from build123d import *

# Parameters (mm, degrees)
F1_DEPTH = 25.4
F2_R     = 3.96875
F3_DEPTH = 25.908


with BuildPart() as f1:
    # F0 (on Front) → F1 (new body)
    with BuildSketch(Plane.XZ):
        with BuildLine():
            add(Edge.make_bspline(
                [(-38.1, -12.7), (-33.882107, -9.031354), (-25.392182, -1.693309), (-12.704204, 19.473612), (0.008999, -0.001138), (12.668207, -19.469058), (25.518173, 1.677371), (33.612126, 9.065506), (38.1, 12.7)],
                knots=[0, 0, 0, 0, 17.960512, 35.921024, 53.881537, 71.842049, 89.802561, 107.763073, 107.763073, 107.763073, 107.763073], degree=3))
            Line((-38.1, -12.7), (-38.1, -30.40595))
            add(Edge.make_bspline(
                [(-38.1, -30.40595), (-33.882107, -26.737304), (-25.392182, -19.399258), (-12.704204, 1.767662), (0.008999, -17.707088), (12.668207, -37.175008), (25.518173, -16.028579), (33.612126, -8.640444), (38.1, -5.00595)],
                knots=[0, 0, 0, 0, 17.960512, 35.921024, 53.881537, 71.842049, 89.802561, 107.763073, 107.763073, 107.763073, 107.763073], degree=3))
            Line((38.1, -5.00595), (38.1, 12.7))
        make_face()
    extrude(amount=F1_DEPTH)

    # F2 (on Top) → F3 (cut, symmetric)
    with BuildSketch(Plane.XY):
        with Locations((-11.43, -12.550292)):
            Circle(F2_R)
    extrude(amount=F3_DEPTH, both=True, mode=Mode.SUBTRACT)


solid = f1.part
Design review of the part built by this model. Coordinates are the model's own, in mm. Coordinates: 2 decimals unless noted, no trailing zeros. Use a Markdown table: item, result.
(1) Wall thickness on probe 1 along Y at (x, z) = (-11.43, 8); probe 2 along X at (y, z) = (-16.75, -11.5); probe 3 along X at (y, z) = (-2.75, -11): over which ranges is each line inside the solid? List them lowest first.
Worked answers:
| item | result |
|---|---|
| probe 1 | y = -25.4 to -16.52, -8.58 to 0 |
| probe 2 | x = -36.72 to -20.71, -4.21 to 9.15, 15.69 to 30.83 |
| probe 3 | x = -36.15 to -20.32, -4.58 to 8.49, 16.35 to 31.33 |
(2) Add section A-A (z = -4). Count the separate pieces of the cut face and the enclosed holes in it, then the cut area to 3 significant figures.
Worked answers:
| item | result |
|---|---|
| separate pieces | 2 |
| enclosed holes | 1 |
| area | 1,150 mm2 |
(3) For P1, Ø4, axis at x = -6, y = -21.5, coming from the -Z side; P2, Ø3, axis at x = 9, y = -8.5, coming from the -Z side; P3, Ø2, axis at x = 24.5, y = -5.5, coming from the -Z side; P4, Ø10, axis at x = 30, z = -24.5, coming from the -Y side, all flat-tipped, find the tip position at first contact; note any pin that passes through.
Worked answers:
| item | result |
|---|---|
| P1 | stops at z = -11.78 |
| P2 | stops at z = -29.98 |
| P3 | stops at z = -20.23 |
| P4 | passes through |
(4) Draft analysis for pull direction X (two halves, no side actions). For faces 1 (the flat face through (38.1, -13, 4)), 2 (the cylindrical face through (-9.6, -16.07, 2.68)), 3 (the flat face through (0, -25.4, -7)), state which applies: released by +X, released by -X, zero draft, split by the parting line, or undercut.
Worked answers:
| item | result |
|---|---|
| face 1 | released by +X |
| face 2 | undercut |
| face 3 | zero draft |
